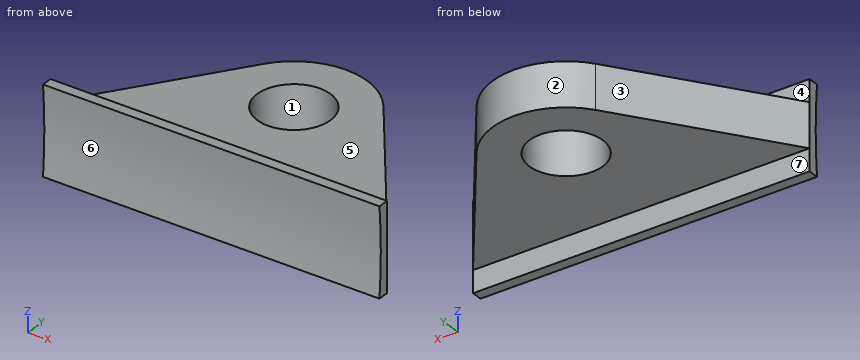
Autodesk Inventor part; units mm, degrees
ref_plane "YZ Plane" through (0, 0, 0) normal (1, 0, 0) x (0, 1, 0)
ref_plane "XZ Plane" through (0, 0, 0) normal (0, 1, 0) x (-1, 0, 0)
ref_plane "XY Plane" through (0, 0, 0) normal (0, 0, 1) x (1, 0, 0)
sketch "Sketch1" plane through (0, 0, 0) normal (0, 0, 1) x (1, 0, 0)
  line L0 (0, 0) -> (-57, 0)
  line L1 (0, 0) -> (58, 0)
  circle A0 centre (0, 40) radius 12.5
  arc A1 (20.1852, 54.7498) -> (-20.3716, 54.4913) centre (0, 40) ccw
  line L2 (-57, 0) -> (-57, 3)
  line L3 (-57, 3) -> (-20.3716, 54.4913)
  line L4 (58, 0) -> (58, 3)
  line L5 (58, 3) -> (20.1852, 54.7498)
  line L6 (-57, 3) -> (58, 3)
  point P0 (29, 0)
  dimension "d0" = 57
  dimension "d1" = 58
  dimension "d3" = 25
  dimension "d4" = 50
  dimension "d5" = 40
  dimension "d6" = 3
  dimension "d7" = 3
extrude "Extrusion1" add sketch "Sketch1" along normal mid plane 15 contours L3 A1 L5 L6
sketch "Sketch2" plane through (0, 0, 0) normal (0, 0, 1) x (1, 0, 0)
  line L0 (-57, 3) -> (58, 3)
  line L1 (-57, 3) -> (-57, 0)
  line L2 (-57, 0) -> (58, 0)
  line L3 (58, 0) -> (58, 3)
  point P0 (0, 0)
  point P1 (0.5, 0)
extrude "Extrusion2" add sketch "Sketch2" along normal mid plane 30
sketch "Sketch3" plane through (58, 0, 15) normal (1, 0, 0) x (0, 0, -1)
  arc A0 (30, -0.6339) -> (0, -0.6339) centre (15, -177.8) ccw
  line L0 (0, 0) -> (30, 0)
  line L1 (30, 0) -> (30, -0.6339)
  line L2 (0, 0) -> (0, -0.6339)
  point P0 (15, 0)
  point P1 (15, 0)
  dimension "d13" = 355.6
extrude "Extrusion3" add sketch "Sketch3" against normal up to surface (115 mm away)
properties part number "Lifting Lug" material "Steel ASTM A36"
CAD build for the part. Positions are in the model's coordinates, mm. Face numbers are marked on the shaded views. A direction names the side the tool comes from. Coordinates: 2 decimals unless noted, no trailing zeros. Order: outer loops, then holes, each group sorted by start corner. A loop starts at its lowest first (then second) coordinate and runs counter-clockwise, first axis right, second up. Notation, with made-up numbers: (32, -30.5) - (80, -30.5) arc R19 ccw to (80, -16.5) - close; hole circle Ø6 at (86.5, 48). An arc over 180 degrees is marked (long way). Answer in a Markdown table with one row per item.
1. Slice it at B-B, the plane y = 32.5. List the corners of the cut face in (x, z), then the cut area to 3 significant figures.
Answer:
| item | result |
|---|---|
| outline | (-36.02, -7.5) - (-10, -7.5) - (-10, 7.5) - (-36.02, 7.5) - close; (10, -7.5) - (36.44, -7.5) - (36.44, 7.5) - (10, 7.5) - close |
| area | 787 mm² |
2. Flat gauge pins, fed straight in: P1, Ø1, axis at x = 26, y = 43.5, coming from the -Z side; P2, Ø2, axis at x = -42, z = -3, coming from the +Y side; P3, Ø5, axis at x = -9, z = 8, coming from the -Y side. Where does each tip first touch, or does it go through?
Answer:
| item | result |
|---|---|
| P1 | z = -7.5 |
| P2 | y = 25.49 |
| P3 | y = -0.31 |
3. Slice it at A-A, the plane x = 0. List the corners of the cut face in (y, z).
Answer:
| item | result |
|---|---|
| outline | (-0.63, -15) - (3, -15) - (3, -7.5) - (27.5, -7.5) - (27.5, 7.5) - (3, 7.5) - (3, 15) - (-0.63, 15) arc R177.8 cw to start; (52.5, -7.5) - (65, -7.5) - (65, 7.5) - (52.5, 7.5) - close |
4. Pull direction X, two halves, no side cores. Call the marked faces 1, 2, 3 and 4: +X half, -X half, draft (parallel to the pull), parting line (faces both ways), or undercut.
Answer:
| item | result |
|---|---|
| face 1 | undercut |
| face 2 | parting line |
| face 3 | -X half |
| face 4 | draft |
5. Slice it at C-C, the plane x = -39. List the corners of the cut face in (y, z), then the cut area to 3 significant figures.
Answer:
| item | result |
|---|---|
| outline | (-0.63, -15) - (3, -15) - (3, -7.5) - (28.3, -7.5) - (28.3, 7.5) - (3, 7.5) - (3, 15) - (-0.63, 15) arc R177.8 cw to start |
| area | 476 mm² |
6. 3-axis set-ups, long thin cutter, end or side, ignore diameter. For the marked faces 5, 6 and 7: which of +Z, -Z, +X, -X, +Y, -Y reach the whole face in a straight line?
Answer:
| item | result |
|---|---|
| face 5 | +Z, +X, -X, +Y |
| face 6 | +X, -X, -Y |
| face 7 | -Z, +X, -X, +Y |
7. Drill centre lines: L1, parallel to Y at x = 0, z = 2; L2, parallel to Z at x = 32, y = 11.5; L3, parallel to X at y = 34.5, z = -2.5. Where is each one in solid material? Low to high. Write a range as from..to.
Answer:
| item | result |
|---|---|
| L1 | -0.01..27.5, 52.5..65 |
| L2 | -7.5..7.5 |
| L3 | -34.59..-11.22, 11.22..34.98 |
8. Slice it at D-D, the plane y = 48. List the corners of the cut face in (x, z).
Answer:
| item | result |
|---|---|
| outline | (-24.99, -7.5) - (-9.6, -7.5) - (-9.6, 7.5) - (-24.99, 7.5) - close; (9.6, -7.5) - (25.12, -7.5) - (25.12, 7.5) - (9.6, 7.5) - close |
